```python
from build123d import *

# Parameters (mm, degrees)
F0_R     = 9.708725
F1_DEPTH = 27.178
F2_R     = 14.948312
F2_R_2   = 9.708725
F3_DEPTH = 10.668


with BuildPart() as f1:
    # F0 (on Front) → F1 (new body)
    with BuildSketch(Plane.XZ):
        Polygon((34.074262, 26.681835), (-30.666837, 26.681835), (-32.127164, -22.300858), (34.074262, -22.300858), align=None)
        Circle(F0_R, mode=Mode.SUBTRACT)
    extrude(amount=F1_DEPTH)

    # F2 (on face) → F3 (join)
    with BuildSketch(Plane.XZ.offset(27.178)):
        Circle(F2_R)
        Circle(F2_R_2, mode=Mode.SUBTRACT)
    extrude(amount=F3_DEPTH)


solid = f1.part
```
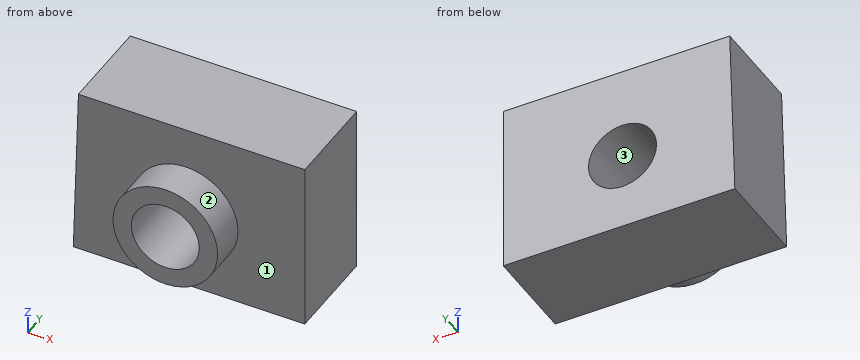
Geometry check sheet. Reference: the model listing, model coordinates, mm. Face numbers are marked on the shaded views. Coordinates: 2 decimals unless noted, no trailing zeros. Loops run counter-clockwise (first coordinate to the right, second up) from the corner with the lowest first, then second, coordinate; pieces in that order, holes last.
Item 1: Sectioned sample at C-C, the plane y = -22. Record the boundary of the cut face in (x, z), then the cut area to 3 significant figures.
Item 2: Release check for a two-part mould opening along Z. For the marked faces 1, 2 and 3 record: released by +Z, released by -Z, zero draft, split by the parting line, or undercut.
Item 3: Go/stop test with flat-tipped pins: pin 1 Ø3 at (x, y) = (5.5, -30.5) entering from +Z; pin 2 Ø8 at (y, z) = (-14, -15) entering from -X. Record where each tip stops, or that it passes through.
Item 4: Sectioned sample at A-A, the plane x = 0. Record the boundary of the cut face in (y, z).
Item 5: Sectioned sample at D-D, the plane x = -27.5. Record the boundary of the cut face in (y, z), then the cut area to 3 significant figures.
Item 6: Sectioned sample at B-B, the plane z = 0. Record the boundary of the cut face in (x, y).
Item 7: Thickness scan on line 1 (Z direction, x = 0, y = -29); line 2 (Z direction, x = 0, y = -11.5); line 3 (Y direction, x = -14, z = 9). Record the ranges inside material, lowest first.
Check result:
1. outline: (-32.13, -22.3) - (34.07, -22.3) - (34.07, 26.68) - (-30.67, 26.68) - close; hole circle Ø19.42 at (0, 0)
1. area: 2,910 mm2
2. face 1: zero draft
2. face 2: split by the parting line
2. face 3: undercut
3. pin 1: stops at z = 14.4
3. pin 2: stops at x = -32.03
4. outline: (-37.85, -14.95) - (-27.18, -14.95) - (-27.18, -22.3) - (0, -22.3) - (0, -9.71) - (-37.85, -9.71) - close; (-37.85, 9.71) - (0, 9.71) - (0, 26.68) - (-27.18, 26.68) - (-27.18, 14.95) - (-37.85, 14.95) - close
5. outline: (-27.18, -22.3) - (0, -22.3) - (0, 26.68) - (-27.18, 26.68) - close
5. area: 1,330 mm2
6. outline: (-31.46, -27.18) - (-14.95, -27.18) - (-14.95, -37.85) - (-9.71, -37.85) - (-9.71, 0) - (-31.46, 0) - close; (9.71, -37.85) - (14.95, -37.85) - (14.95, -27.18) - (34.07, -27.18) - (34.07, 0) - (9.71, 0) - close
7. line 1: z = -14.95 to -9.71, 9.71 to 14.95
7. line 2: z = -22.3 to -9.71, 9.71 to 26.68
7. line 3: y = -27.18 to 0
